Could you check a few things on this model? Use its own coordinates, in mm. Face numbers are marked on the shaded views. A direction names the side the tool comes from. Round coordinates to 2 decimals unless told otherwise and drop trailing zeros. Write each loop counter-clockwise with the first axis right and the second up, starting at its lowest first coordinate (ties: lowest second). Pieces come first, ordered by that corner, then holes. Notation, with made-up numbers: (-36.5, 68) - (-28.5, 68) arc R14 cw to (-28.5, 94) - close; hole circle Ø5 at (-4.75, -17). An arc over 180 degrees is marked (long way). Put each result on its own line as item: value.
from build123d import *

# Parameters (mm, degrees)
F0_W     = 60
F0_H     = 60
F1_DEPTH = 5
F0_R     = 45
F2_DEPTH = 15
F4_DEPTH = 4
F5_DEPTH = 7


# Not quite as in the source:
# - a fillet or chamfer that OpenCascade refuses, or shapes differently, is made with other operations: its cross-section is extruded or revolved along the edge and cut away or added


with BuildPart() as f1:
    # F0 (on Top) → F1 (new body)
    with BuildSketch(Plane.XY):
        Rectangle(F0_W, F0_H)
        with BuildLine():
            Line((25, 24), (25, 0))
            Line((25, 0), (25, -24))
            ThreePointArc((25, -24), (25.7071067812, -24.2928932188), (26, -25))
            ThreePointArc((26, -25), (25, -26), (24, -25))
            Line((24, -25), (-5.83e-08, -25))
            Line((-5.83e-08, -25), (-24, -25))
            ThreePointArc((-24, -25), (-25.7071067812, -25.7071067812), (-25, -24))
            Line((-25, -24), (-25, 2.61e-08))
            Line((-25, 2.61e-08), (-25, 24))
            ThreePointArc((-25, 24), (-25.7071067812, 25.7071067812), (-24, 25))
            Line((-24, 25), (0, 25))
            Line((0, 25), (24, 25))
            ThreePointArc((24, 25), (25, 26), (26, 25))
            ThreePointArc((26, 25), (25.7071067812, 24.2928932188), (25, 24))
        make_face(mode=Mode.SUBTRACT)
        with BuildLine():
            ThreePointArc((0, 25), (17.6776695297, 17.6776695297), (25, 0))
            Line((25, 0), (25, 24))
            ThreePointArc((25, 24), (24.2928932188, 24.2928932188), (24, 25))
            Line((24, 25), (0, 25))
        make_face()
        with BuildLine():
            Line((30, 30), (30, -30))
            ThreePointArc((30, -30), (39.1968889463, -16.2358830044), (42.4264068712, 0))
            ThreePointArc((42.4264068712, 0), (39.1968889463, 16.2358830044), (30, 30))
        make_face()
        with BuildLine():
            ThreePointArc((-30, -30), (0, -42.4264068712), (30, -30))
            Line((30, -30), (-30, -30))
        make_face()
        with BuildLine():
            ThreePointArc((-30, 30), (-42.4264068712, 0), (-30, -30))
            Line((-30, -30), (-30, 30))
        make_face()
        with BuildLine():
            Line((-24, -25), (-5.83e-08, -25))
            ThreePointArc((-5.83e-08, -25), (-17.6776695595, -17.6776694998), (-25, 2.61e-08))
            Line((-25, 2.61e-08), (-25, -24))
            ThreePointArc((-25, -24), (-24.2928932188, -24.2928932188), (-24, -25))
        make_face()
        with BuildLine():
            Line((25, -24), (25, 0))
            ThreePointArc((25, 0), (17.677669509, -17.6776695503), (-5.83e-08, -25))
            Line((-5.83e-08, -25), (24, -25))
            ThreePointArc((24, -25), (24.2928932188, -24.2928932188), (25, -24))
        make_face()
        with BuildLine():
            ThreePointArc((-25, 2.61e-08), (-17.6776695204, 17.6776695389), (0, 25))
            Line((0, 25), (-24, 25))
            ThreePointArc((-24, 25), (-24.2928932188, 24.2928932188), (-25, 24))
            Line((-25, 24), (-25, 2.61e-08))
        make_face()
        with BuildLine():
            Line((-30, 30), (30, 30))
            ThreePointArc((30, 30), (0, 42.4264068712), (-30, 30))
        make_face()
    extrude(amount=F1_DEPTH)

    # F0 (on Top) → F2 (join)
    with BuildSketch(Plane.XY):
        Circle(F0_R)
        with BuildLine():
            ThreePointArc((42.4264068712, 0), (39.1968889463, -16.2358830044), (30, -30))
            ThreePointArc((30, -30), (0, -42.4264068712), (-30, -30))
            ThreePointArc((-30, -30), (-42.4264068712, 0), (-30, 30))
            ThreePointArc((-30, 30), (0, 42.4264068712), (30, 30))
            ThreePointArc((30, 30), (39.1968889463, 16.2358830044), (42.4264068712, 0))
        make_face(mode=Mode.SUBTRACT)
    extrude(amount=F2_DEPTH)

    # F3: chamfer of 5 on 1 edges, made by hand

    # F3_s1 → F3_t2 (revolve, cut)
    with BuildSketch(Plane.XZ):
        Polygon((40, 15), (45, 10), (45, 15), align=None)
    revolve(axis=Axis((0, 0, 15), (0, 0, 1)), mode=Mode.SUBTRACT)

    # F0 (on Top) → F4 (join)
    with BuildSketch(Plane.XY):
        Circle(F0_R)
        with BuildLine():
            ThreePointArc((42.4264068712, 0), (39.1968889463, -16.2358830044), (30, -30))
            ThreePointArc((30, -30), (0, -42.4264068712), (-30, -30))
            ThreePointArc((-30, -30), (-42.4264068712, 0), (-30, 30))
            ThreePointArc((-30, 30), (0, 42.4264068712), (30, 30))
            ThreePointArc((30, 30), (39.1968889463, 16.2358830044), (42.4264068712, 0))
        make_face(mode=Mode.SUBTRACT)
    extrude(amount=-F4_DEPTH)

    # F0 (on Top) → F5 (join)
    with BuildSketch(Plane.XY):
        Circle(F0_R)
        with BuildLine():
            ThreePointArc((42.4264068712, 0), (39.1968889463, -16.2358830044), (30, -30))
            ThreePointArc((30, -30), (0, -42.4264068712), (-30, -30))
            ThreePointArc((-30, -30), (-42.4264068712, 0), (-30, 30))
            ThreePointArc((-30, 30), (0, 42.4264068712), (30, 30))
            ThreePointArc((30, 30), (39.1968889463, 16.2358830044), (42.4264068712, 0))
        make_face(mode=Mode.SUBTRACT)
    extrude(amount=-F5_DEPTH)


solid = f1.part
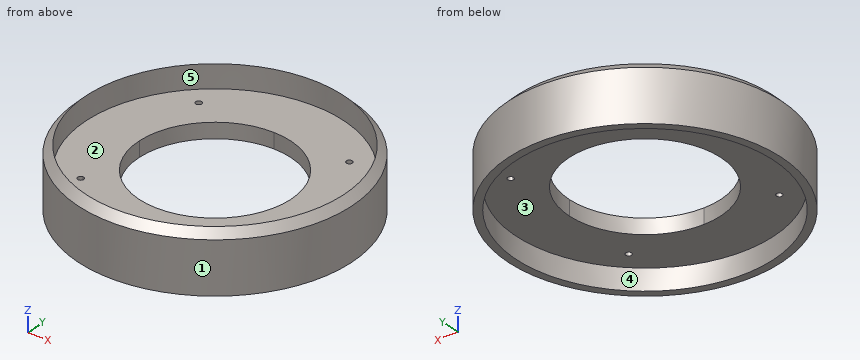
(1) For the marked faces 4 and 5, which set-ups out of +Z, -Z, +X, -X, +Y, -Y let a thin tool reach every point of the face, with its end or its side?
Values found:
face 4: -Z
face 5: +Z
(2) Imagine slicing it at A-A, the plane z = -1.5. List the corners of the cut face in (x, y) for me.
Values found:
outline: circle Ø90 at (0, 0); hole circle Ø84.85 at (0, 0)
(3) Please list where these lines run through material, in increasing order: probe 1 along Z at (x, y) = (39, -9); probe 2 along X at (y, z) = (-2.5, 3.75); probe 3 along Y at (x, z) = (-6.5, -3). Write a range as from..to.
Values found:
probe 1: z = 0..5
probe 2: x = -44.93..-24.87, 24.87..44.93
probe 3: y = -44.53..-41.93, 41.93..44.53
(4) If we mould it in two halves opening along Y, with no side actions, what happens to the marked faces 1, 2 and 3? For each: pulls with the +Y half, pulls with the -Y half, needs draft (parallel to the pull), parting line crosses it, or undercut.
Values found:
face 1: parting line crosses it
face 2: undercut
face 3: undercut
(5) I'm going to push flat-ended pins straight in: pin 1 (2.5 mm diameter, centred on x = -25, y = 25, fed in from +Z); pin 2 (1 mm diameter, centred on y = -17.5, z = 8.5, fed in from -X); pin 3 (5 mm diameter, centred on x = 8, z = -2.5, fed in from -Y); pin 4 (1.6 mm diameter, centred on x = -25, y = -25, fed in from -Z). Where does each tip first touch, or does it pass through?
Values found:
pin 1: stops at z = 5
pin 2: stops at x = -41.67
pin 3: stops at y = -44.66
pin 4: passes through
